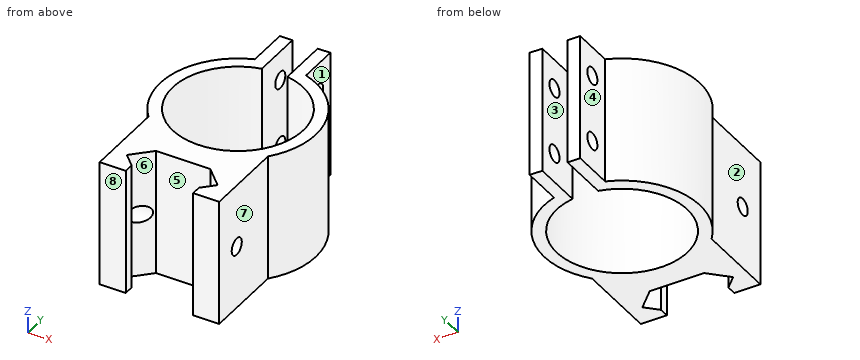
```python
from build123d import *

# Parameters (mm, degrees)
BOSS_EXTRUDE1_DEPTH = 30
SKETCH2_R           = 2
CUT_EXTRUDE1_DEPTH  = 25.140587276
SKETCH3_R           = 2
CUT_EXTRUDE2_DEPTH  = 33.7


with BuildPart() as part:
    # Sketch1 → Boss-Extrude1 (new body)
    with BuildSketch(Plane.XY):
        with BuildLine():
            Line((2.640587276, 55.058478526), (2.640587276, 61.071909479))
            Line((2.640587276, 61.071909479), (5.640587276, 61.071909479))
            Line((5.640587276, 61.071909479), (5.640587276, 51.377039696))
            ThreePointArc((5.640587276, 51.377039696), (17.766153021, 38.916765877), (14.2, 21.9))
            Line((14.2, 21.9), (14.2, 2.5))
            Line((14.2, 2.5), (11.082842712, 2.5))
            Line((11.082842712, 2.5), (8, 2.5))
            Line((8, 2.5), (8, 4.817157288))
            Line((8, 4.817157288), (10.782842712, 7.6))
            Line((10.782842712, 7.6), (6.482842712, 11.9))
            Line((6.482842712, 11.9), (-6.482842712, 11.9))
            Line((-6.482842712, 11.9), (-10.782842712, 7.6))
            Line((-10.782842712, 7.6), (-8, 4.817157288))
            Line((-8, 4.817157288), (-8, 2.5))
            Line((-8, 2.5), (-11.082842712, 2.5))
            Line((-11.082842712, 2.5), (-14.2, 2.5))
            Line((-14.2, 2.5), (-14.2, 21.9))
            ThreePointArc((-14.2, 21.9), (-17.868360087, 38.550789704), (-6.359412724, 51.130527146))
            Line((-6.359412724, 51.130527146), (-6.359412724, 61.069189213))
            Line((-6.359412724, 61.069189213), (-3.359412724, 61.069189213))
            Line((-3.359412724, 61.069189213), (-3.359412724, 55.069189213))
            Line((-3.359412724, 55.069189213), (-3.359412724, 48.889476621))
            ThreePointArc((-3.359412724, 48.889476621), (0.366343929, 18.262238644), (2.640587276, 49.0313268))
            Line((2.640587276, 49.0313268), (2.640587276, 55.058478526))
        make_face()
    extrude(amount=BOSS_EXTRUDE1_DEPTH)

    # Sketch2 → Cut-Extrude1 (cut, through all)
    with BuildSketch(Plane(origin=(5.640587276, 0, 0), x_dir=(0, 0, -1), z_dir=(1, 0, 0))):
        with Locations(Location((-7, 56.224474587, 0), (0, 0, 270))):  # turned: the seam where the file's is
            Circle(SKETCH2_R)
        with Locations(Location((-23, 56.224474587, 0), (0, 0, 270))):  # turned: the seam where the file's is
            Circle(SKETCH2_R)
    extrude(amount=-CUT_EXTRUDE1_DEPTH, mode=Mode.SUBTRACT)

    # Sketch3 → Cut-Extrude2 (cut, through all)
    with BuildSketch(Plane(origin=(14.2, 0, 0), x_dir=(0, 0, -1), z_dir=(1, 0, 0))):
        with Locations(Location((-15, 9.5, 0), (0, 0, 90))):  # turned: the seam where the file's is
            Circle(SKETCH3_R)
    extrude(amount=-CUT_EXTRUDE2_DEPTH, mode=Mode.SUBTRACT)


solid = part.part
```
Model file for the job. Use its own axes, mm. Face numbers are marked on the shaded views. A direction names the side the tool comes from. Give positions to 0.01 mm unless a question says otherwise; leave off trailing zeros. Order: outer loops, then holes, each group sorted by start corner. A loop starts at its lowest first (then second) coordinate and runs counter-clockwise, first axis right, second up.
1) Mould opens along Y. For the marked faces 6, 7 and 8 say: +Y half, -Y half, draft (parallel to the pull), parting line (faces both ways), or undercut.
2) Saw through at A-A, the plane z = 7. Write the cut outline in (x, y), then the cut area to 3 significant figures.
3) Pin check, flat tips, straight feed: pin 1 (3 mm diameter, centred on y = 58, z = 11.5, fed in from -X); pin 2 (2.5 mm diameter, centred on y = 56.22, z = 23, fed in from +X); pin 3 (1 mm diameter, centred on x = -8, z = 5.5, fed in from +Y); pin 4 (6 mm diameter, centred on y = 8, z = 17.5, fed in from +X). Stop position of each tip, or through.
4) Saw through at C-C, the plane y = 9.5. Write the cut outline in (x, z).
5) Wall check: probe 1 along X at (y, z) = (56, 12.5); probe 2 along Y at (x, z) = (12, 15); probe 3 along Y at (x, z) = (-4.45, 7). Give the ranges that are in metal, low to high.
6) Saw through at B-B, the plane x = -13. Write the cut outline in (y, z), then the cut area to 3 significant figures.
7) Saw through at D-D, the plane z = 10.5. Write the cut outline in (x, y), then the cut area to 3 significant figures.
8) 3-axis set-ups, long thin cutter, end or side, ignore diameter. For the marked faces 1, 2, 3, 4 and 5: which of +Z, -Z, +X, -X, +Y, -Y reach the whole face in a straight line?
Computed:
1. face 6: undercut
1. face 7: draft
1. face 8: -Y half
2. outline: (-14.2, 2.5) - (-8, 2.5) - (-8, 4.82) - (-10.78, 7.6) - (-6.48, 11.9) - (6.48, 11.9) - (10.78, 7.6) - (8, 4.82) - (8, 2.5) - (14.2, 2.5) - (14.2, 21.9) arc R18.5 ccw to (5.64, 51.38) - (5.64, 54.22) - (2.64, 54.22) - (2.64, 49.03) arc R15.5 cw (long way) to (-3.36, 48.89) - (-3.36, 54.22) - (-6.36, 54.22) - (-6.36, 51.13) arc R18.5 ccw to (-14.2, 21.9) - close; (-6.36, 58.22) - (-3.36, 58.22) - (-3.36, 61.07) - (-6.36, 61.07) - close; (2.64, 58.22) - (5.64, 58.22) - (5.64, 61.07) - (2.64, 61.07) - close
2. area: 591 mm2
3. pin 1: stops at x = -6.36
3. pin 2: passes through
3. pin 3: stops at y = 50.67
3. pin 4: stops at x = 14.2
4. outline: (-14.2, 0) - (-8.88, 0) - (-8.88, 13) - (-14.2, 13) - close; (-14.2, 17) - (-8.88, 17) - (-8.88, 30) - (-14.2, 30) - close; (8.88, 0) - (14.2, 0) - (14.2, 13) - (8.88, 13) - close; (8.88, 17) - (14.2, 17) - (14.2, 30) - (8.88, 30) - close
5. probe 1: x = -6.36 to -3.36, 2.64 to 5.64
5. probe 2: y = 2.5 to 7.5, 11.5 to 23.95, 43.57 to 47.84
5. probe 3: y = 11.9 to 18.91, 48.61 to 54.22, 58.22 to 61.07
6. outline: (2.5, 0) - (25.32, 0) - (25.32, 30) - (2.5, 30) - close; (42.2, 0) - (46.92, 0) - (46.92, 30) - (42.2, 30) - close; hole circle Ø4 at (9.5, 15)
6. area: 814 mm2
7. outline: (-14.2, 2.5) - (-8, 2.5) - (-8, 4.82) - (-10.78, 7.6) - (-6.48, 11.9) - (6.48, 11.9) - (10.78, 7.6) - (8, 4.82) - (8, 2.5) - (14.2, 2.5) - (14.2, 21.9) arc R18.5 ccw to (5.64, 51.38) - (5.64, 61.07) - (2.64, 61.07) - (2.64, 49.03) arc R15.5 cw (long way) to (-3.36, 48.89) - (-3.36, 61.07) - (-6.36, 61.07) - (-6.36, 51.13) arc R18.5 ccw to (-14.2, 21.9) - close
7. area: 615 mm2
8. face 1: +Z, -Z, +X, +Y
8. face 2: +Z, -Z, -X, -Y
8. face 3: +Z, -Z, +Y
8. face 4: +Z, -Z, -X, +Y
8. face 5: +Z, -Z, -Y
